Here's how the part is built. I have some questions about the finished solid (model axes, mm). A direction names the side the tool comes from. Coordinates: 2 decimals unless noted, no trailing zeros. Write each loop counter-clockwise with the first axis right and the second up, starting at its lowest first coordinate (ties: lowest second). Pieces come first, ordered by that corner, then holes.
(1) Imagine slicing it at B-B, the plane x = 0. List the corners of the cut face in (y, z) for me.
(2) Thinking about a two-plate mould opening in Z: for faces 1 (the cylindrical face through (-0.97, 3.55, -1.27)), 2 (the cylindrical face through (17.86, 3.45, 5.83)), 3 (the cylindrical face through (4.49, 3.45, -7.8)), which applies, released by +Z, released by -Z, zero draft, split by the parting line, or undercut?
(3) For pin 1 Ø5 at (x, z) = (-112, 0) entering from -Y; pin 2 Ø3 at (x, y) = (7, 3) entering from +Z; pin 3 Ø1.5 at (x, y) = (-16, 0.5) entering from +Z; pin 4 Ø2 at (x, y) = (-89.5, 6) entering from -Z, each with a flat end and sliding along its axis, tell me the tip position at first contact or that it passes through.
(4) Imagine slicing it at A-A, the plane x = 36. List the corners of the cut face in (y, z) for me.
(5) Please list where these lines run through material, in increasing order: probe 1 along X at (y, z) = (2.25, 1.75); probe 2 along Z at (x, y) = (-96, 4.25); probe 3 along Z at (x, y) = (-94.5, 1).
(6) Which directions (+Z, -Z, +X, -X, +Y, -Y) give clear straight access to the entire face, cutting with the end or side of a thin tool? Please do faces 4 (the cylindrical face through (-120, 3, 0)), 5 (the flat face through (19, 3, 0)).
(7) Imagine slicing it at C-C, the plane y = 4. List the corners of the cut face in (x, z) for me, plus the area to 3 significant figures.
(8) Imagine slicing it at D-D, the plane x = -64. List the corners of the cut face in (y, z) for me.
```python
from build123d import *

# Parameters (mm, degrees)
SKETCH1_R           = 2
SKETCH1_R_2         = 1.6
BOSS_EXTRUDE1_DEPTH = 7
SKETCH4_R           = 1.6
CUT_EXTRUDE1_DEPTH  = 10


with BuildPart() as part:
    # Sketch1 → Boss-Extrude1 (new body)
    with BuildSketch(Plane(origin=(0, 0, 0), x_dir=(1, 0, 0), z_dir=(0, 1, 0))):
        with BuildLine():
            ThreePointArc((-110.092216302, 7.769193096), (-120, 0), (-110.092216302, -7.769193096))
            ThreePointArc((-110.092216302, -7.769193096), (-57.431509927, -1.988156982), (-4.756803809, -7.640210568))
            ThreePointArc((-4.756803809, -7.640210568), (0, -9), (4.756803809, -7.640210568))
            ThreePointArc((4.756803809, -7.640210568), (18.044616959, -5.824262713), (31.43520243, -6.569826721))
            ThreePointArc((31.43520243, -6.569826721), (43.089371642, 3.706859819), (28, 0))
            Line((28, 0), (9, 0))
            ThreePointArc((9, 0), (4.369711988, 7.868012274), (-4.756803809, 7.640210568))
            ThreePointArc((-4.756803809, 7.640210568), (-57.431509927, 1.988156982), (-110.092216302, 7.769193096))
        make_face()
        with Locations(Location((-112, 0, 0), (0, 0, 270))):
            Circle(SKETCH1_R, mode=Mode.SUBTRACT)
        with Locations(Location((36, 0, 0), (0, 0, 270))):
            Circle(SKETCH1_R_2, mode=Mode.SUBTRACT)
    extrude(amount=BOSS_EXTRUDE1_DEPTH)

    # Sketch4 → Cut-Extrude1 (cut)
    with BuildSketch(Plane(origin=(0, 7, 0), x_dir=(1, 0, 0), z_dir=(0, 1, 0))):
        with Locations(Location((0, 0, 0), (0, 0, 270))):
            Circle(SKETCH4_R)
    extrude(amount=-CUT_EXTRUDE1_DEPTH, mode=Mode.SUBTRACT)


solid = part.part
```
Recorded:
1. outline: (0, -9) - (7, -9) - (7, -1.6) - (0, -1.6) - close; (0, 1.6) - (7, 1.6) - (7, 9) - (0, 9) - close
2. face 1: undercut
2. face 2: released by +Z
2. face 3: released by -Z
3. pin 1: stops at y = 0
3. pin 2: stops at z = 7.47
3. pin 3: stops at z = 5.59
3. pin 4: stops at z = -4.27
4. outline: (0, -8) - (7, -8) - (7, -1.6) - (0, -1.6) - close; (0, 1.6) - (7, 1.6) - (7, 8) - (0, 8) - close
5. probe 1: x = -119.81 to -112.97, -111.03 to 43.81
5. probe 2: z = -5.08 to 5.08
5. probe 3: z = -4.85 to 4.85
6. face 4: +Y, -Y
6. face 5: -Z, +Y, -Y
7. outline: (-110.09, -7.77) arc R245.48 cw to (-4.76, -7.64) arc R9 ccw to (9, 0) - (28, 0) arc R8 ccw (long way) to (31.44, 6.57) arc R70.16 cw to (4.76, 7.64) arc R9 ccw to (-4.76, 7.64) arc R245.48 cw to (-110.09, 7.77) arc R8 ccw (long way) to start; hole circle Ø4 at (-112, 0); hole circle Ø3.2 at (0, 0); hole circle Ø3.2 at (36, 0)
7. area: 1,460 mm2
8. outline: (0, -2.08) - (7, -2.08) - (7, 2.08) - (0, 2.08) - close
